The drawing under review shows one solid part. Ordinate dimensions are in mm from its lowest x, y, z. Coordinates: 2 decimals unless noted, no trailing zeros. Write each loop counter-clockwise with the first axis right and the second up, starting at its lowest first coordinate (ties: lowest second). Pieces come first, ordered by that corner, then holes. Notation, with made-up numbers: (-27, 3.25) -> (-20, 3.25) arc R19 ccw to (-20, 19.25) -> close; hole circle Ø11 at (6.5, -4). An arc over 180 degrees is marked (long way). Put each result on its own line as item: value. Start each with the question number.
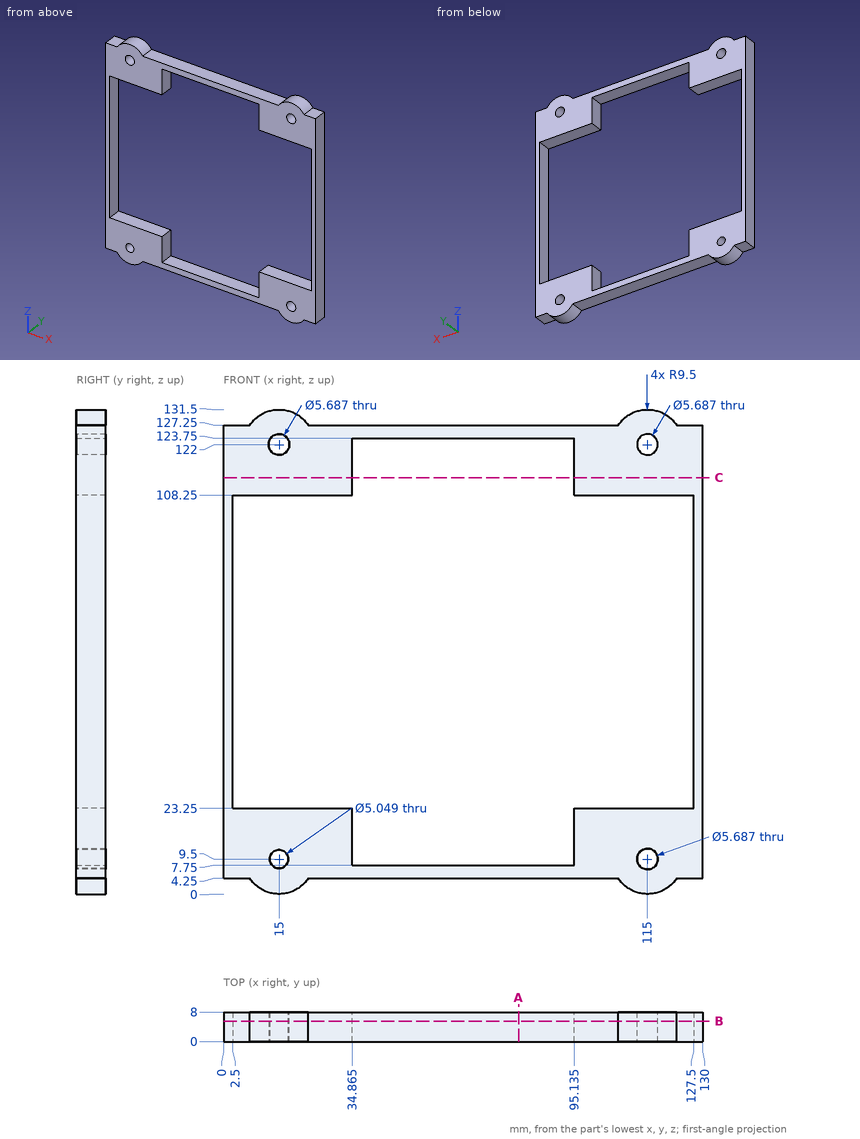
1. Wall thickness on line 1 (Z direction, x = 115, y = 3.75); line 2 (X direction, y = 4, z = 18) (1 decimal); line 3 (X direction, y = 2.5, z = 9.5) (1 decimal): over which ranges is each line inside the solid? List them lowest first. Write a range as from..to.
2. Consider section C-C on z = 113. State the section outline as (x, y) points (1 decimal), then the cut area to 3 significant figures.
3. Insertion check: P1, Ø10, axis at x = 83.5, z = 16, coming from the +Y side; P2, Ø4, axis at x = 68, y = 2, coming from the +Z side; P3, Ø7.5, axis at x = 115, z = 122, coming from the +Y side; P4, Ø1, axis at x = 23, y = 3.5, coming from the -Z side. Each pin has a flat end and moves straight along its axis. Give the tip position at first contact, or say it passes through.
4. Consider section A-A on x = 80. State the section outline as (y, z) points.
5. Consider section B-B on y = 5.5. State how many separate pieces and enclosed holes the cut face has, then the cut area to 3 significant figures.
Output values:
1. line 1: z = 0..6.66, 12.34..23.25, 108.25..119.16, 124.84..131.5
1. line 2: x = 0..34.9, 95.1..130
1. line 3: x = 0..12.5, 17.5..34.9, 95.1..112.2, 117.8..130
2. outline: (0, 0) -> (34.9, 0) -> (34.9, 8) -> (0, 8) -> close; (95.1, 0) -> (130, 0) -> (130, 8) -> (95.1, 8) -> close
2. area: 558 mm^2
3. P1: passes through
3. P2: stops at z = 127.25
3. P3: stops at y = 8
3. P4: stops at z = 3.67
4. outline: (0, 4.25) -> (8, 4.25) -> (8, 7.75) -> (0, 7.75) -> close; (0, 123.75) -> (8, 123.75) -> (8, 127.25) -> (0, 127.25) -> close
5. separate pieces: 1
5. enclosed holes: 5
5. area: 3,590 mm^2
